from build123d import *

# Parameters (mm, degrees)
BOSS_EXTRUDE1_DEPTH     = 3
SKETCH2_R               = 1.5
CUT_EXTRUDE1_DEPTH      = 4
CUT_EXTRUDE1_DEPTH_BACK = 4
SKETCH3_R               = 3
CUT_EXTRUDE2_DEPTH      = 4
CUT_EXTRUDE2_DEPTH_BACK = 4


with BuildPart() as part:
    # Sketch1 → Boss-Extrude1 (new body, symmetric)
    with BuildSketch(Plane(origin=(0, 0, 0), x_dir=(0, 0, -1), z_dir=(1, 0, 0))):
        with BuildLine():
            Line((40, -10), (0, -10))
            ThreePointArc((0, -10), (-10, 0), (0, 10))
            Line((0, 10), (40, 10))
            ThreePointArc((40, 10), (50, 0), (40, -10))
        make_face()
    extrude(amount=BOSS_EXTRUDE1_DEPTH, both=True)

    # Sketch2 → Cut-Extrude1 (cut, two sides)
    with BuildSketch(Plane(origin=(0, 0, 0), x_dir=(0, 0, -1), z_dir=(1, 0, 0))) as cut_extrude1_sk:
        with Locations((4.949747468, 4.949747468)):
            Circle(SKETCH2_R)
        with Locations((4.949747468, -4.949747468)):
            Circle(SKETCH2_R)
        with Locations((-4.949747468, -4.949747468)):
            Circle(SKETCH2_R)
        with Locations((-4.949747468, 4.949747468)):
            Circle(SKETCH2_R)
    extrude(amount=CUT_EXTRUDE1_DEPTH, mode=Mode.SUBTRACT)
    extrude(cut_extrude1_sk.sketch, amount=-CUT_EXTRUDE1_DEPTH_BACK, mode=Mode.SUBTRACT)

    # Sketch3 → Cut-Extrude2 (cut, two sides)
    with BuildSketch(Plane(origin=(0, 0, 0), x_dir=(0, 0, -1), z_dir=(1, 0, 0))) as cut_extrude2_sk:
        with Locations((40, 0)):
            Circle(SKETCH3_R)
    extrude(amount=CUT_EXTRUDE2_DEPTH, mode=Mode.SUBTRACT)
    extrude(cut_extrude2_sk.sketch, amount=-CUT_EXTRUDE2_DEPTH_BACK, mode=Mode.SUBTRACT)


solid = part.part
Design review of the part built by this model. Coordinates are the model's own, in mm. Coordinates: 2 decimals unless noted, no trailing zeros. Order: outer loops, then holes, each group sorted by start corner. A loop starts at its lowest first (then second) coordinate and runs counter-clockwise, first axis right, second up.
Item 1: Take a section at A-A, the plane y = 0. Write out the cut boundary in (x, z).
Item 2: For pin 1 Ø2.5 at (y, z) = (4.95, -4.95) entering from +X; pin 2 Ø1 at (x, y) = (-0.5, -8) entering from +Z, all flat-tipped, find the tip position at first contact; note any pin that passes through.
Item 3: Take a section at D-D, the plane z = -46. Write out the cut boundary in (x, y), then the cut area to 3 significant figures.
Item 4: For line 1 (Y direction, x = 0.8, z = -40); line 2 (Z direction, x = -1.8, y = -5.5); line 3 (Y direction, x = 1.8, z = 6), list the stretches that pass through material, from the lowest coordinate up.
Item 5: Take a section at B-B, the plane z = 5.5. Write out the cut boundary in (x, y), then the cut area to 3 significant figures.
Item 6: Take a section at C-C, the plane x = -2.4. Write out the cut boundary in (y, z).
Item 7: The part is to be moulded in two halves that separate along Y. For faces 1 (the flat face through (0, 10, -20)), 2 (the cylindrical face through (0, 0, -37)), 3 (the cylindrical face through (0, 0, -50)), 4 (the cylindrical face through (0.04, 4.04, 6.14)), say which applies: pulls with the +Y half, pulls with the -Y half, needs draft (parallel to the pull), parting line crosses it, or undercut.
The answers:
1. outline: (-3, -50) - (3, -50) - (3, -43) - (-3, -43) - close; (-3, -37) - (3, -37) - (3, 10) - (-3, 10) - close
2. pin 1: passes through
2. pin 2: stops at z = 6.61
3. outline: (-3, -8) - (3, -8) - (3, 8) - (-3, 8) - close
3. area: 96.0 mm2
4. line 1: y = -10 to -3, 3 to 10
4. line 2: z = -48.35 to -6.35, -3.55 to 3.55, 6.35 to 8.35
4. line 3: y = -8 to -6.02, -3.88 to 3.88, 6.02 to 8
5. outline: (-3, -8.35) - (3, -8.35) - (3, -6.35) - (-3, -6.35) - close; (-3, -3.55) - (3, -3.55) - (3, 3.55) - (-3, 3.55) - close; (-3, 6.35) - (3, 6.35) - (3, 8.35) - (-3, 8.35) - close
5. area: 66.7 mm2
6. outline: (-10, -40) arc R10 ccw to (10, -40) - (10, 0) arc R10 ccw to (-10, 0) - close; hole circle Ø3 at (-4.95, -4.95); hole circle Ø3 at (-4.95, 4.95); hole circle Ø6 at (0, -40); hole circle Ø3 at (4.95, -4.95); hole circle Ø3 at (4.95, 4.95)
7. face 1: pulls with the +Y half
7. face 2: undercut
7. face 3: parting line crosses it
7. face 4: undercut
